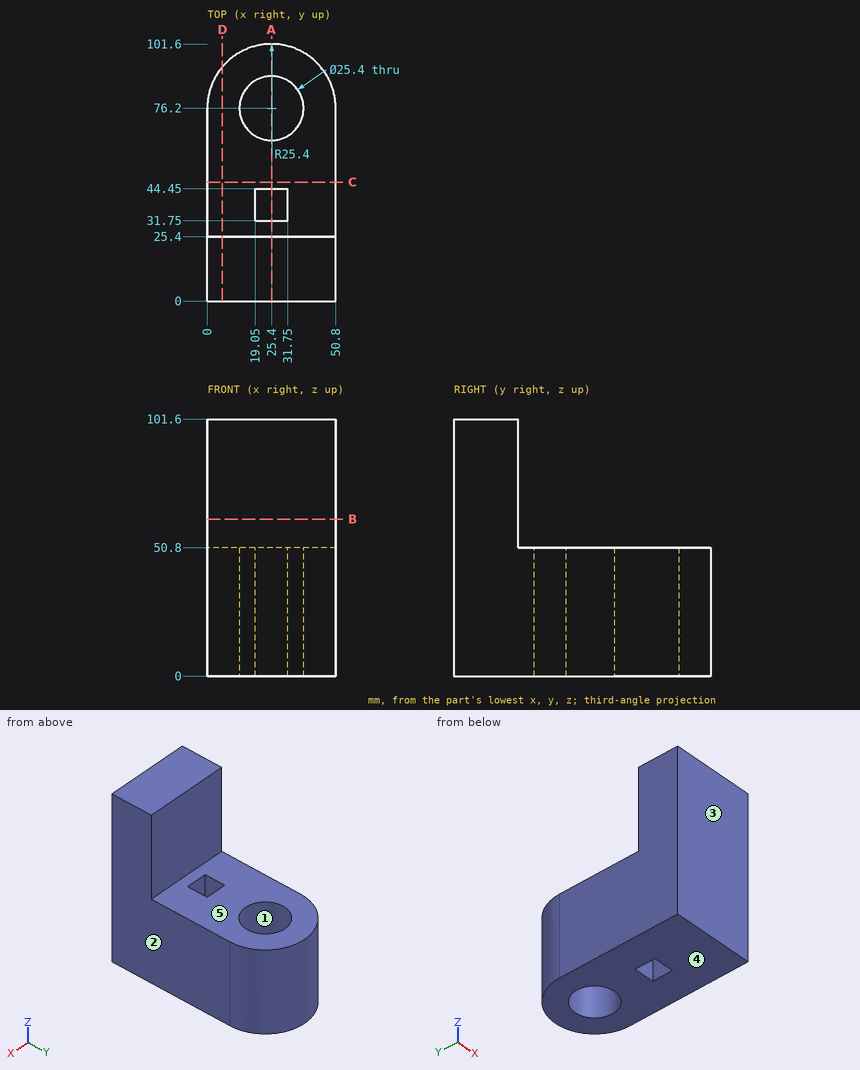
Here's the drawing with two shaded views (mm, measured from the low corner). I have some questions. A direction names the side the tool comes from. Coordinates: 2 decimals unless noted, no trailing zeros. Loops run counter-clockwise (first coordinate to the right, second up) from the corner with the lowest first, then second, coordinate; pieces in that order, holes last. Notation, with made-up numbers: M 61,-6 L 93,-6 A18 ccw 93,14 Z; hole C -15,15.5 d3. An arc over 180 degrees is marked long. Return JSON: item names as keys, results as strings. Group by question number.
Item 1: If I drill on L1, parallel to Y at x = 25.4, z = 30.5; L2, parallel to X at y = 76, z = 11; L3, parallel to Y at x = 21, z = 41, over which ranges is the centre line in solid material (lowest first)? Write a range as from..to.
Item 2: Imagine slicing it at C-C (y = 47). Please give me the cut outline in (x, z).
Item 3: I'm going to push flat-ended pins straight in: pin 1 Ø4 at (x, z) = (22.5, 18) entering from +Y; pin 2 Ø8 at (x, z) = (16.5, 58.5) entering from +Y; pin 3 Ø8 at (x, z) = (40.5, 46) entering from +Y; pin 4 Ø3 at (x, y) = (24.5, 86) entering from -Z. Where does each tip first touch, or does it pass through?
Item 4: Imagine slicing it at A-A (x = 25.4). Please give me the cut outline in (y, z), and give its area (3 significant figures).
Item 5: Thinking about a two-plate mould opening in Y: for the marked faces 1, 2 and 3, which applies, released by +Y, released by -Y, zero draft, split by the parting line, or undercut?
Item 6: Imagine slicing it at D-D (x = 6). Please give me the cut outline in (y, z), and give its area (3 significant figures).
Item 7: On a 3-axis mill with a long thin cutter (end or side, diameter ignored), from which of +Z, -Z, +X, -X, +Y, -Y can I reach the whole of each face in a straight line? I mean the marked faces 4 and 5. Say none if no direction works.
Item 8: Imagine slicing it at B-B (z = 62). Please give me the cut outline in (x, y).
Verdict:
{
 "1": {"L1": "y = 0..31.75, 44.45..63.5, 88.9..101.6", "L2": "x = 0..12.7, 38.1..50.8", "L3": "y = 0..31.75, 44.45..64.29, 88.11..101.22"},
 "2": {"outline": "M 0,0 L 50.8,0 L 50.8,50.8 L 0,50.8 Z"},
 "3": {"pin 1": "stops at y = 101.58", "pin 2": "stops at y = 25.4", "pin 3": "stops at y = 99.05", "pin 4": "passes through"},
 "4": {"outline": "M 0,0 L 31.75,0 L 31.75,50.8 L 25.4,50.8 L 25.4,101.6 L 0,101.6 Z; M 44.45,0 L 63.5,0 L 63.5,50.8 L 44.45,50.8 Z; M 88.9,0 L 101.6,0 L 101.6,50.8 L 88.9,50.8 Z", "area": "4,520 mm^2"},
 "5": {"face 1": "undercut", "face 2": "zero draft", "face 3": "released by -Y"},
 "6": {"outline": "M 0,0 L 92.6,0 L 92.6,50.8 L 25.4,50.8 L 25.4,101.6 L 0,101.6 Z", "area": "5,990 mm^2"},
 "7": {"face 4": "-Z, +X, -X, +Y, -Y", "face 5": "+Z, +X, -X, +Y"},
 "8": {"outline": "M 0,0 L 50.8,0 L 50.8,25.4 L 0,25.4 Z"}
}
